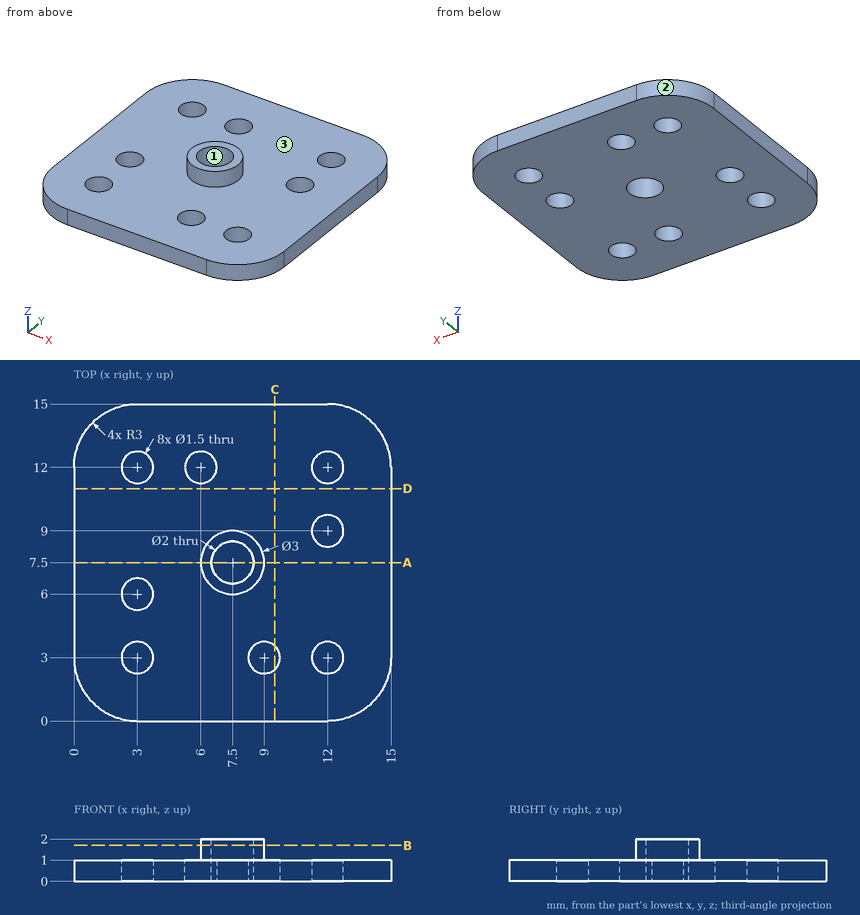
Part print with two shaded views. Sizes in mm from the minimum x, y, z corner. Round coordinates to 2 decimals unless told otherwise and drop trailing zeros. Order: outer loops, then holes, each group sorted by start corner. A loop starts at its lowest first (then second) coordinate and runs counter-clockwise, first axis right, second up. Notation, with made-up numbers: (61, 34) - (105, 34) arc R32 cw to (105, 73) - close; hole circle Ø2 at (-29, 68). An arc over 180 degrees is marked (long way). Answer in a Markdown table with one row per item. Add a question column.
(1) Mould opens along Y. For the marked faces 1, 2 and 3 say: +Y half, -Y half, draft (parallel to the pull), parting line (faces both ways), or undercut.
(2) Drop flat-ended pins along their axis: pin 1 Ø1.2 at (x, y) = (3, 3) entering from -Z; pin 2 Ø2 at (x, y) = (4, 11.5) entering from +Z. Give the stop position or say it passes through.
(3) Band-saw the part on A-A on y = 7.5. List the corners of the cut face in (x, z), and give its area (3 significant figures).
(4) Band-saw the part on C-C on x = 9.5. List the corners of the cut face in (y, z).
(5) Band-saw the part on B-B on z = 1.7. List the corners of the cut face in (x, y), and give its area (3 significant figures).
(6) Probe L1, parallel to X at y = 9, z = 0.5; L2, parallel to Y at x = 12.5, z = 0.9. List the from-to ranges inside material, lowest first. Write a range as [from, to].
(7) Band-saw the part on D-D on y = 11. List the corners of the cut face in (x, z).
Data:
| question | item | result |
|---|---|---|
| 1 | face 1 | undercut |
| 1 | face 2 | +Y half |
| 1 | face 3 | draft |
| 2 | pin 1 | passes through |
| 2 | pin 2 | stops at z = 1 |
| 3 | outline | (0, 0) - (6.5, 0) - (6.5, 2) - (6, 2) - (6, 1) - (0, 1) - close; (8.5, 0) - (15, 0) - (15, 1) - (9, 1) - (9, 2) - (8.5, 2) - close |
| 3 | area | 14.0 mm^2 |
| 4 | outline | (0, 0) - (2.44, 0) - (2.44, 1) - (0, 1) - close; (3.56, 0) - (15, 0) - (15, 1) - (3.56, 1) - close |
| 5 | outline | circle Ø3 at (7.5, 7.5); hole circle Ø2 at (7.5, 7.5) |
| 5 | area | 3.93 mm^2 |
| 6 | L1 | x = [0, 11.25], [12.75, 15] |
| 6 | L2 | y = [0.04, 2.44], [3.56, 8.44], [9.56, 11.44], [12.56, 14.96] |
| 7 | outline | (0, 0) - (15, 0) - (15, 1) - (0, 1) - close |
